Can you work these out from the model? Positions are in its coordinate system, mm. Face numbers are marked on the shaded views. A direction names the side the tool comes from. Give positions to 0.01 mm unless a question says otherwise; leave off trailing zeros. Order: outer loops, then holes, each group sorted by start corner. A loop starts at its lowest first (then second) coordinate and runs counter-clockwise, first axis right, second up. Notation, with made-up numbers: (9.25, -6) -> (68.25, -6) arc R34 ccw to (68.25, 29) -> close; hole circle Ø7 at (-3, 44.5). An arc over 180 degrees is marked (long way). Answer as a JSON object with one key per item and string values.
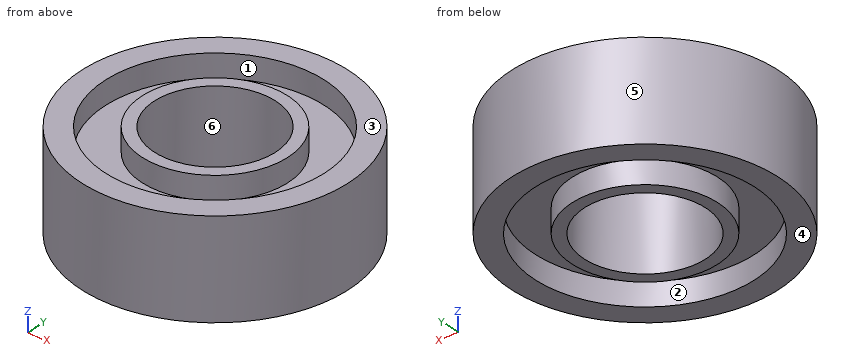
```python
from build123d import *

# Parameters (mm, degrees)
SKETCH1_R           = 5.5
SKETCH1_R_2         = 2.5
BOSS_EXTRUDE1_DEPTH = 2
SKETCH2_R           = 4.526057725
SKETCH2_R_2         = 3.002990226
CUT_EXTRUDE1_DEPTH  = 0.952


with BuildPart() as part:
    # Sketch1 → Boss-Extrude1 (new body)
    with BuildSketch(Plane.XY):
        Circle(SKETCH1_R)
        Circle(SKETCH1_R_2, mode=Mode.SUBTRACT)
    extrude(amount=BOSS_EXTRUDE1_DEPTH)

    # Sketch2 → Cut-Extrude1 (cut)
    with BuildSketch(Plane.XY.offset(2)):
        Circle(SKETCH2_R)
        Circle(SKETCH2_R_2, mode=Mode.SUBTRACT)
    extrude(amount=-CUT_EXTRUDE1_DEPTH, mode=Mode.SUBTRACT)

    # Mirror1: part across plane


with BuildPart() as part_1:
    add(part.part)
    add(part.part.mirror(Plane.XY))


solid = part_1.part
```
1. If we section it at D-D on y = -2.75: Please give me the cut outline in (x, z), then the cut area to 3 significant figures.
Worked answers:
{"outline": "(-4.76, -2) -> (-3.59, -2) -> (-3.59, -1.05) -> (-1.21, -1.05) -> (-1.21, -2) -> (1.21, -2) -> (1.21, -1.05) -> (3.59, -1.05) -> (3.59, -2) -> (4.76, -2) -> (4.76, 2) -> (3.59, 2) -> (3.59, 1.05) -> (1.21, 1.05) -> (1.21, 2) -> (-1.21, 2) -> (-1.21, 1.05) -> (-3.59, 1.05) -> (-3.59, 2) -> (-4.76, 2) -> close", "area": "29.0 mm²"}
2. Please list where these lines run through material, in increasing order: L1, parallel to Y at x = 0, z = 1.15; L2, parallel to Y at x = 0, z = 0.95; L3, parallel to X at y = 2, z = -1.5.
Worked answers:
{"L1": "-5.5 to -4.53, -3 to -2.5, 2.5 to 3, 4.53 to 5.5", "L2": "-5.5 to -2.5, 2.5 to 5.5", "L3": "-5.12 to -4.06, -2.24 to -1.5, 1.5 to 2.24, 4.06 to 5.12"}
3. If we mould it in two halves opening along Y, with no side actions, what happens to the marked faces 4, 5 and 6? For each: +Y half, -Y half, draft (parallel to the pull), parting line (faces both ways), or undercut.
Worked answers:
{"face 4": "draft", "face 5": "parting line", "face 6": "undercut"}
4. If we section it at A-A on x = 0: Please give me the cut outline in (y, z), then the cut area to 3 significant figures.
Worked answers:
{"outline": "(-5.5, -2) -> (-4.53, -2) -> (-4.53, -1.05) -> (-3, -1.05) -> (-3, -2) -> (-2.5, -2) -> (-2.5, 2) -> (-3, 2) -> (-3, 1.05) -> (-4.53, 1.05) -> (-4.53, 2) -> (-5.5, 2) -> close; (2.5, -2) -> (3, -2) -> (3, -1.05) -> (4.53, -1.05) -> (4.53, -2) -> (5.5, -2) -> (5.5, 2) -> (4.53, 2) -> (4.53, 1.05) -> (3, 1.05) -> (3, 2) -> (2.5, 2) -> close", "area": "18.2 mm²"}
5. Will this pin go through, and if not, where does the flat tip stop? pin 1 Ø1.5 at (y, z) = (3, -0.5) entering from -X.
Worked answers:
{"pin 1": "x = -5.02"}
6. If we section it at B-B on y = -1.5: Please give me the cut outline in (x, z), then the cut area to 3 significant figures.
Worked answers:
{"outline": "(-5.29, -2) -> (-4.27, -2) -> (-4.27, -1.05) -> (-2.6, -1.05) -> (-2.6, -2) -> (-2, -2) -> (-2, 2) -> (-2.6, 2) -> (-2.6, 1.05) -> (-4.27, 1.05) -> (-4.27, 2) -> (-5.29, 2) -> close; (2, -2) -> (2.6, -2) -> (2.6, -1.05) -> (4.27, -1.05) -> (4.27, -2) -> (5.29, -2) -> (5.29, 2) -> (4.27, 2) -> (4.27, 1.05) -> (2.6, 1.05) -> (2.6, 2) -> (2, 2) -> close", "area": "20.0 mm²"}
7. For the marked faces 1, 2 and 3, which set-ups out of +Z, -Z, +X, -X, +Y, -Y let a thin tool reach every point of the face, with its end or its side?
Worked answers:
{"face 1": "+Z", "face 2": "-Z", "face 3": "+Z, +X, -X, +Y, -Y"}
8. If we section it at C-C on y = 3.75: Please give me the cut outline in (x, z), then the cut area to 3 significant figures.
Worked answers:
{"outline": "(-4.02, -2) -> (-2.53, -2) -> (-2.53, -1.05) -> (2.53, -1.05) -> (2.53, -2) -> (4.02, -2) -> (4.02, 2) -> (2.53, 2) -> (2.53, 1.05) -> (-2.53, 1.05) -> (-2.53, 2) -> (-4.02, 2) -> close", "area": "22.5 mm²"}
